```python
from build123d import *

# Parameters (mm, degrees)
SKETCH1_W           = 27
SKETCH1_H           = 17
SKETCH1_W_2         = 23
SKETCH1_H_2         = 13
BOSS_EXTRUDE1_DEPTH = 18
SKETCH1_2_W         = 27
SKETCH1_2_H         = 17
SKETCH1_2_W_2       = 23
SKETCH1_2_H_2       = 13
BOSS_EXTRUDE2_DEPTH = 2
SKETCH2_R           = 1.5
CUT_EXTRUDE1_DEPTH  = 2
SKETCH3_W           = 10
SKETCH3_H           = 5
CUT_EXTRUDE2_DEPTH  = 3
SKETCH4_W           = 4
SKETCH4_H           = 17
BOSS_EXTRUDE3_DEPTH = 3
SKETCH5_R           = 1
CUT_EXTRUDE3_DEPTH  = 5


with BuildPart() as part:
    # Sketch1 → Boss-Extrude1 (new body)
    with BuildSketch(Plane(origin=(0, 0, 0), x_dir=(1, 0, 0), z_dir=(0, 1, 0))):
        Rectangle(SKETCH1_W, SKETCH1_H)
        Rectangle(SKETCH1_W_2, SKETCH1_H_2, mode=Mode.SUBTRACT)
    extrude(amount=BOSS_EXTRUDE1_DEPTH)

    # Sketch1_2 → Boss-Extrude2 (add)
    # profile 1 of 2: a face of its own
    with BuildSketch(Plane(origin=(0, 0, 0), x_dir=(1, 0, 0), z_dir=(0, 1, 0))):
        Rectangle(SKETCH1_2_W, SKETCH1_2_H)
        Rectangle(SKETCH1_2_W_2, SKETCH1_2_H_2, mode=Mode.SUBTRACT)
    # profile 2 of 2: a face of its own
    with BuildSketch(Plane(origin=(0, 0, 0), x_dir=(1, 0, 0), z_dir=(0, 1, 0))):
        Rectangle(SKETCH1_2_W_2, SKETCH1_2_H_2)
    extrude(amount=-BOSS_EXTRUDE2_DEPTH)

    # Sketch2 → Cut-Extrude1 (cut)
    with BuildSketch(Plane(origin=(0, 0, 0), x_dir=(1, 0, 0), z_dir=(0, 1, 0))):
        with Locations(Location((-6, 0, 0), (0, 0, 270))):
            Circle(SKETCH2_R)
        with Locations(Location((0, 0, 0), (0, 0, 270))):
            Circle(SKETCH2_R)
        with Locations(Location((6, 0, 0), (0, 0, 270))):
            Circle(SKETCH2_R)
    extrude(amount=-CUT_EXTRUDE1_DEPTH, mode=Mode.SUBTRACT)

    # Sketch3 → Cut-Extrude2 (cut)
    with BuildSketch(Plane.ZY.offset(13.5)):
        with Locations((0, 6.5)):
            Rectangle(SKETCH3_W, SKETCH3_H)
    extrude(amount=-CUT_EXTRUDE2_DEPTH, mode=Mode.SUBTRACT)

    # Sketch4 → Boss-Extrude3 (add)
    with BuildSketch(Plane(origin=(0, 18, 0), x_dir=(1, 0, 0), z_dir=(0, 1, 0))):
        with Locations((15.5, 0)):
            Rectangle(SKETCH4_W, SKETCH4_H)
        with Locations((-15.5, 0)):
            Rectangle(SKETCH4_W, SKETCH4_H)
    extrude(amount=-BOSS_EXTRUDE3_DEPTH)

    # Sketch5 → Cut-Extrude3 (cut)
    with BuildSketch(Plane(origin=(0, 18, 0), x_dir=(1, 0, 0), z_dir=(0, 1, 0))):
        with Locations(Location((-13.5, 0, 0), (0, 0, 270))):
            Circle(SKETCH5_R)
        with Locations(Location((13.5, 0, 0), (0, 0, 270))):
            Circle(SKETCH5_R)
    extrude(amount=-CUT_EXTRUDE3_DEPTH, mode=Mode.SUBTRACT)


solid = part.part
```
For this review, take the finished solid that the model builds, in its own axes (mm). A direction names the side the tool comes from. Round coordinates to 2 decimals unless told otherwise and drop trailing zeros. Loops run counter-clockwise (first coordinate to the right, second up) from the corner with the lowest first, then second, coordinate; pieces in that order, holes last.
Q1. Add section A-A on z = -4.5. Write out the cut boundary in (x, y).
Result sheet:
outline: (-17.5, 15) - (-13.5, 15) - (-13.5, 9) - (-11.5, 9) - (-11.5, 18) - (-17.5, 18) - close; (-13.5, -2) - (13.5, -2) - (13.5, 15) - (17.5, 15) - (17.5, 18) - (11.5, 18) - (11.5, 0) - (-11.5, 0) - (-11.5, 4) - (-13.5, 4) - close
Q2. Mouldability with a two-part tool opening along Z and no side actions: class faces 6 (the face through (0, 8, 8.5)), 7 (the face through (-12.51, 16.09, -0.13)), 8 (the face through (-7.33, -0.99, 0.69)), 9 (the face through (17.5, 17, 0)) as +Z half, -Z half, draft (parallel to the pull), parting line (faces both ways), or undercut.
Result sheet:
face 6: +Z half
face 7: undercut
face 8: undercut
face 9: draft
Q3. Add section C-C on y = 11. Write out the cut boundary in (x, z).
Result sheet:
outline: (-13.5, -8.5) - (13.5, -8.5) - (13.5, 8.5) - (-13.5, 8.5) - close; hole (-11.5, -6.5) - (11.5, -6.5) - (11.5, 6.5) - (-11.5, 6.5) - close
Q4. Add section D-D on y = 6.5. Write out the cut boundary in (x, z), plus the area to 3 significant figures.
Result sheet:
outline: (-13.5, -8.5) - (13.5, -8.5) - (13.5, 8.5) - (-13.5, 8.5) - (-13.5, 5) - (-11.5, 5) - (-11.5, 6.5) - (11.5, 6.5) - (11.5, -6.5) - (-11.5, -6.5) - (-11.5, -5) - (-13.5, -5) - close
area: 140 mm2
Q5. Machinability: for faces 1 (the face through (12.61, 16.09, 0.46)), 2 (the face through (-13.5, 3, 0)), 3 (the face through (0, 8, -8.5)), 4 (the face through (0, -2, -2)), 5 (the face through (-13, 6, -5)), which of the approach directions +Z, -Z, +X, -X, +Y, -Y give a long, thin tool a straight path to every point of the face, cutting with its end or side? Answer none if there is none.
Result sheet:
face 1: +Y
face 2: +Z, -Z, -X, -Y
face 3: -Z, +X, -X, +Y, -Y
face 4: +Z, -Z, +X, -X, -Y
face 5: -X
Q6. Add section B-B on x = 0. Write out the cut boundary in (y, z), plus the area to 4 significant figures.
Result sheet:
outline: (-2, -8.5) - (18, -8.5) - (18, -6.5) - (0, -6.5) - (0, -1.5) - (-2, -1.5) - close; (-2, 1.5) - (0, 1.5) - (0, 6.5) - (18, 6.5) - (18, 8.5) - (-2, 8.5) - close
area: 100.0 mm2
Q7. Insertion check: pin 1 Ø1.2 at (x, z) = (-15, -0.5) entering from -Y; pin 2 Ø1.8 at (x, z) = (-6, 0) entering from +Y; pin 3 Ø1 at (y, z) = (0.5, 2) entering from -X; pin 4 Ø0.5 at (x, z) = (13, 0.5) entering from +Y. Each pin has a flat end and moves straight along its axis. Give the tip position at first contact, or say it passes through.
Result sheet:
pin 1: stops at y = 15
pin 2: passes through
pin 3: stops at x = -13.5
pin 4: stops at y = 13
Q8. To check wall thickness, follow line 1 along X through (y, z) = (-1.3, 0); line 2 along Z through (x, y) = (-7, 8.25); line 3 along X through (y, z) = (15.75, 0). State the ranges of each line that lie inside material, in increasing order.
Result sheet:
line 1: x = -13.5 to -7.5, -4.5 to -1.5, 1.5 to 4.5, 7.5 to 13.5
line 2: z = -8.5 to -6.5, 6.5 to 8.5
line 3: x = -17.5 to -14.5, -12.5 to -11.5, 11.5 to 12.5, 14.5 to 17.5
